Geometry check sheet. Reference: the model listing, model coordinates, mm. A direction names the side the tool comes from. Coordinates: 2 decimals unless noted, no trailing zeros. Order: outer loops, then holes, each group sorted by start corner. A loop starts at its lowest first (then second) coordinate and runs counter-clockwise, first axis right, second up. Notation, with made-up numbers: (57, 86) - (105, 86) arc R18 ccw to (105, 93) - close; hole circle Ø1 at (29, 65). An arc over 180 degrees is marked (long way). Use CSV: the item, a comma, the result in double quotes. Start each with the question number.
1) Sectioned sample at D-D, the plane z = 3.75. Record the cut outline in (x, y).
2) Draft check along X on faces 5 (the flat face through (0, 0.7, 8)), 6 (the cylindrical face through (8.334, 1.547, 7.935)), 7 (the flat face through (-10.5, 0, 8)), 8 (the flat face through (-10, 0.3, 8)). Enter one of: released by +X, released by -X, zero draft, split by the parting line, or undercut.
3) Thickness scan on probe 1 along Y at (x, z) = (-3, 5.75); probe 2 along Z at (x, y) = (-2.5, -0.45); probe 3 along Z at (x, y) = (-4, -1.3). Record the ranges inside material, lowest first. Write a range as [from, to].
4) Sectioned sample at B-B, the plane x = -3.5. Record the cut outline in (y, z), and give its area (3 significant figures).
5) Sectioned sample at A-A, the plane z = 13.75. Record the cut outline in (x, y), and give its area (3 significant figures).
6) Depth check by flat-ended pin: P1, Ø1, axis at x = -9.5, y = -1, coming from the +Z side (3 decimals); P2, Ø0.8, axis at x = -10, z = 8, coming from the +Y side; P3, Ø4, axis at x = -8.5, z = 2.5, coming from the -Y side; P4, Ø2, axis at x = -9, y = -1, coming from the -Z side (3 decimals). Enter the tip coordinate at first touch or a pass-through.
7) Tool access check on faces 1 (the flat face through (-9, -1, 11.175)), 2 (the flat face through (9, 1, 4.825)), 3 (the cylindrical face through (-8, -0.6, 7.9)), 4 (the flat face through (10, -0.3, 8)). Record the directions out of +Z, -Z, +X, -X, +Y, -Y that give a thin tool (end or side, any length) a straight path to the whole face; none if there is none.
8) Sectioned sample at C-C, the plane z = 7.5. Record the cut outline in (x, y).
from build123d import *

# Parameters (mm, degrees)
BOSS_EXTRUDE1_DEPTH     = 16
CUT_EXTRUDE2_DEPTH      = 16
CUT_EXTRUDE2_DEPTH_BACK = 16
SKETCH2_R               = 16.202009592


with BuildPart() as part:
    # Sketch1 → Boss-Extrude1 (new body)
    with BuildSketch(Plane.XY):
        with BuildLine():
            Line((6.5, -1.7), (-6.5, -1.7))
            ThreePointArc((-6.5, -1.7), (-8.359565153, -1.542285751), (-10.166007905, -1.073648442))
            ThreePointArc((-10.166007905, -1.073648442), (-10.408046537, -0.890971778), (-10.5, -0.602011532))
            Line((-10.5, -0.602011532), (-10.5, 0.3))
            Line((-10.5, 0.3), (-9.5, 0.3))
            Line((-9.5, 0.3), (-9.5, -0.3))
            ThreePointArc((-9.5, -0.3), (-8.013274595, -0.599559463), (-6.5, -0.7))
            Line((-6.5, -0.7), (6.5, -0.7))
            ThreePointArc((6.5, -0.7), (6.6, -0.6), (6.5, -0.5))
            Line((6.5, -0.5), (-6.5, -0.5))
            ThreePointArc((-6.5, -0.5), (-7.6, 0.6), (-6.5, 1.7))
            Line((-6.5, 1.7), (6.5, 1.7))
            ThreePointArc((6.5, 1.7), (8.359565153, 1.542285751), (10.166007905, 1.073648442))
            ThreePointArc((10.166007905, 1.073648442), (10.408046537, 0.890971778), (10.5, 0.602011532))
            Line((10.5, 0.602011532), (10.5, -0.3))
            Line((10.5, -0.3), (9.5, -0.3))
            Line((9.5, -0.3), (9.5, 0.3))
            ThreePointArc((9.5, 0.3), (8.013274595, 0.599559463), (6.5, 0.7))
            Line((6.5, 0.7), (-6.5, 0.7))
            ThreePointArc((-6.5, 0.7), (-6.6, 0.6), (-6.5, 0.5))
            Line((-6.5, 0.5), (6.5, 0.5))
            ThreePointArc((6.5, 0.5), (7.6, -0.6), (6.5, -1.7))
        make_face()
    extrude(amount=BOSS_EXTRUDE1_DEPTH)

    # Sketch2 → Cut-Extrude2 (cut, two sides: drawn at the far end of the back side and taken through both)
    # profile 1 of 5: a face of its own
    with BuildSketch(Plane(origin=(0, 1.7, 0), x_dir=(1, 0, 0), z_dir=(0, 1, 0)).offset(-CUT_EXTRUDE2_DEPTH_BACK)):
        with Locations((0, -8)):
            Circle(SKETCH2_R)
        with BuildLine():
            ThreePointArc((-6.5, -12.663689527), (-6.961399446, -11.941943399), (-7.342981343, -11.175))
            Line((-7.342981343, -11.175), (-10.5, -11.175))
            Line((-10.5, -11.175), (-10.5, -4.825))
            Line((-10.5, -4.825), (-7.342981343, -4.825))
            ThreePointArc((-7.342981343, -4.825), (-6.961399446, -4.058056601), (-6.5, -3.336310473))
            Line((-6.5, -3.336310473), (-6.5, 0))
            Line((-6.5, 0), (0, 0))
            Line((0, 0), (6.5, 0))
            Line((6.5, 0), (6.5, -3.336310473))
            ThreePointArc((6.5, -3.336310473), (6.961399446, -4.058056601), (7.342981343, -4.825))
            Line((7.342981343, -4.825), (10.5, -4.825))
            Line((10.5, -4.825), (10.5, -11.175))
            Line((10.5, -11.175), (7.342981343, -11.175))
            ThreePointArc((7.342981343, -11.175), (6.961399446, -11.941943399), (6.5, -12.663689527))
            Line((6.5, -12.663689527), (6.5, -16))
            Line((6.5, -16), (0, -16))
            Line((0, -16), (-6.5, -16))
            Line((-6.5, -16), (-6.5, -12.663689527))
        make_face(mode=Mode.SUBTRACT)
    # profile 2 of 5: a face of its own
    with BuildSketch(Plane(origin=(0, 1.7, 0), x_dir=(1, 0, 0), z_dir=(0, 1, 0)).offset(-CUT_EXTRUDE2_DEPTH_BACK)):
        with BuildLine():
            ThreePointArc((0, -16), (-3.653114, -15.117215615), (-6.5, -12.663689527))
            Line((-6.5, -12.663689527), (-6.5, -16))
            Line((-6.5, -16), (0, -16))
        make_face()
    # profile 3 of 5: a face of its own
    with BuildSketch(Plane(origin=(0, 1.7, 0), x_dir=(1, 0, 0), z_dir=(0, 1, 0)).offset(-CUT_EXTRUDE2_DEPTH_BACK)):
        with BuildLine():
            ThreePointArc((6.5, -12.663689527), (3.653114, -15.117215615), (0, -16))
            Line((0, -16), (6.5, -16))
            Line((6.5, -16), (6.5, -12.663689527))
        make_face()
    # profile 4 of 5: a face of its own
    with BuildSketch(Plane(origin=(0, 1.7, 0), x_dir=(1, 0, 0), z_dir=(0, 1, 0)).offset(-CUT_EXTRUDE2_DEPTH_BACK)):
        with BuildLine():
            Line((-6.5, 0), (-6.5, -3.336310473))
            ThreePointArc((-6.5, -3.336310473), (-3.653114, -0.882784385), (0, 0))
            Line((0, 0), (-6.5, 0))
        make_face()
    # profile 5 of 5: a face of its own
    with BuildSketch(Plane(origin=(0, 1.7, 0), x_dir=(1, 0, 0), z_dir=(0, 1, 0)).offset(-CUT_EXTRUDE2_DEPTH_BACK)):
        with BuildLine():
            Line((6.5, 0), (0, 0))
            ThreePointArc((0, 0), (3.653114, -0.882784385), (6.5, -3.336310473))
            Line((6.5, -3.336310473), (6.5, 0))
        make_face()
    extrude(amount=CUT_EXTRUDE2_DEPTH + CUT_EXTRUDE2_DEPTH_BACK, mode=Mode.SUBTRACT)


solid = part.part
Evaluation:
1,outline,"(-6.78, -1.7) arc R11.04 ccw to (-6.5, -1.7) - (6.5, -1.7) arc R1.1 ccw to (6.78, -1.66) - (6.78, 0.46) arc R1.1 ccw to (6.5, 0.5) - (-6.5, 0.5) arc R0.1 cw to (-6.5, 0.7) - (6.5, 0.7) arc R11.45 cw to (6.78, 0.7) - (6.78, 1.7) arc R11.04 ccw to (6.5, 1.7) - (-6.5, 1.7) arc R1.1 ccw to (-6.78, 1.66) - (-6.78, -0.46) arc R1.1 ccw to (-6.5, -0.5) - (6.5, -0.5) arc R0.1 cw to (6.5, -0.7) - (-6.5, -0.7) arc R11.45 cw to (-6.78, -0.7) - close"
2,face 5,"undercut"
2,face 6,"released by +X"
2,face 7,"released by -X"
2,face 8,"zero draft"
3,probe 1,"[-1.7, -0.7], [-0.5, 0.5], [0.7, 1.7]"
3,probe 2,"[0.4, 15.6]"
3,probe 3,"[1.07, 14.93]"
4,outline,"(-1.7, 0.81) - (-0.7, 0.81) - (-0.7, 15.19) - (-1.7, 15.19) - close; (-0.5, 0.81) - (0.5, 0.81) - (0.5, 15.19) - (-0.5, 15.19) - close; (0.7, 0.81) - (1.7, 0.81) - (1.7, 15.19) - (0.7, 15.19) - close"
4,area,"43.2 mm²"
5,outline,"(-5.56, -1.7) - (5.56, -1.7) - (5.56, -0.7) - (-5.56, -0.7) - close; (-5.56, -0.5) - (5.56, -0.5) - (5.56, 0.5) - (-5.56, 0.5) - close; (-5.56, 0.7) - (5.56, 0.7) - (5.56, 1.7) - (-5.56, 1.7) - close"
5,area,"33.4 mm²"
6,P1,"z = 11.175"
6,P2,"y = 0.3"
6,P3,"through"
6,P4,"z = 4.825"
7,face 1,"+Z, -X, +Y, -Y"
7,face 2,"-Z, +X, +Y, -Y"
7,face 3,"+Z, -Z"
7,face 4,"+Z, -Z, +X, -Y"
8,outline,"(-10.5, -0.6) arc R0.5 ccw to (-10.17, -1.07) arc R11.04 ccw to (-6.5, -1.7) - (6.5, -1.7) arc R1.1 ccw to (6.5, 0.5) - (-6.5, 0.5) arc R0.1 cw to (-6.5, 0.7) - (6.5, 0.7) arc R11.45 cw to (9.5, 0.3) - (9.5, -0.3) - (10.5, -0.3) - (10.5, 0.6) arc R0.5 ccw to (10.17, 1.07) arc R11.04 ccw to (6.5, 1.7) - (-6.5, 1.7) arc R1.1 ccw to (-6.5, -0.5) - (6.5, -0.5) arc R0.1 cw to (6.5, -0.7) - (-6.5, -0.7) arc R11.45 cw to (-9.5, -0.3) - (-9.5, 0.3) - (-10.5, 0.3) - close"
